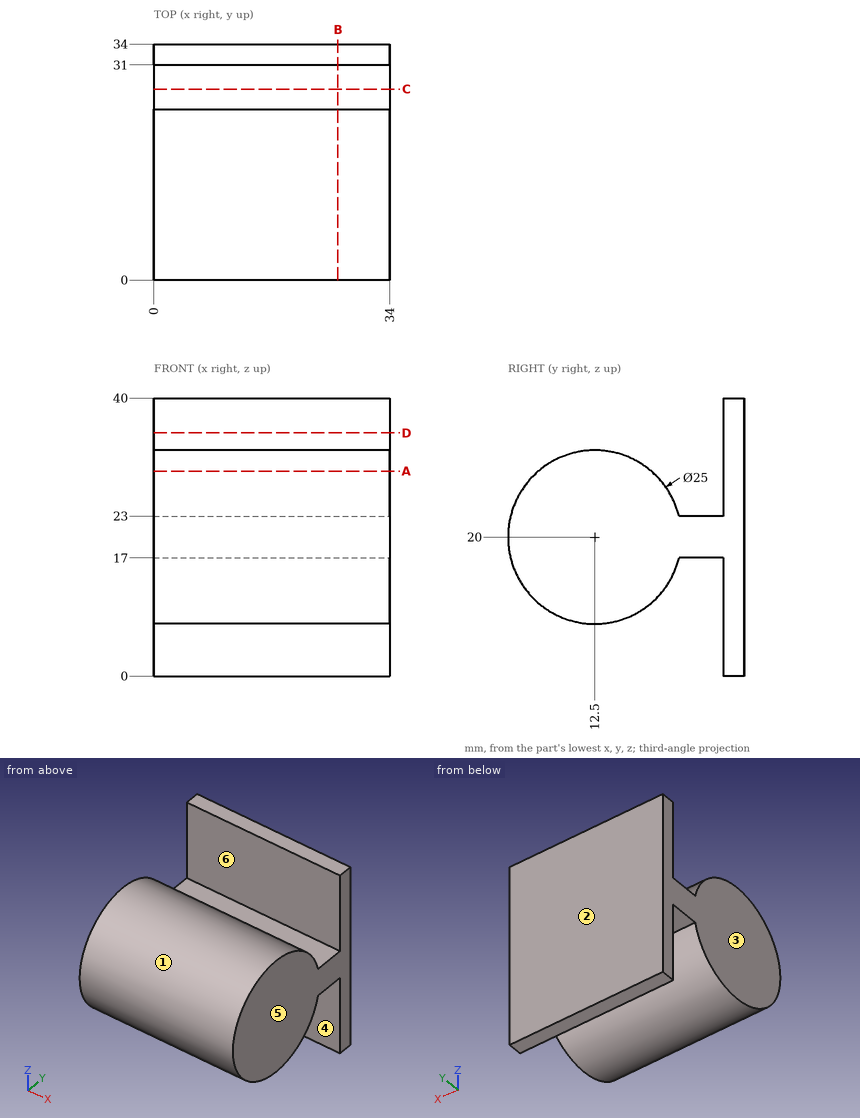
The drawing under review shows one solid part. Ordinate dimensions are in mm from its lowest x, y, z. A direction names the side the tool comes from. Round coordinates to 2 decimals unless told otherwise and drop trailing zeros. Write each loop counter-clockwise with the first axis right and the second up, starting at its lowest first coordinate (ties: lowest second). Pieces come first, ordered by that corner, then holes. Notation, with made-up numbers: (36, 17.5) - (83, 17.5) arc R25 ccw to (83, 55.5) - close; hole circle Ø7 at (-23, 51). An arc over 180 degrees is marked (long way). Put each result on its own line as item: value.
Q1. We need section A-A (z = 29.5). Give the boundary of the cut face in (x, y).
Solved:
outline: (0, 4.38) - (34, 4.38) - (34, 20.62) - (0, 20.62) - close; (0, 31) - (34, 31) - (34, 34) - (0, 34) - close
Q2. We need section D-D (z = 35). Give the boundary of the cut face in (x, y), and give its area (3 significant figures).
Solved:
outline: (0, 31) - (34, 31) - (34, 34) - (0, 34) - close
area: 102 mm2
Q3. Wall thickness on probe 1 along Y at (x, z) = (23.5, 5.5); probe 2 along Z at (x, y) = (2, 29); probe 3 along Z at (x, y) = (16, 13): over which ranges is each line inside the solid? List them lowest first.
Solved:
probe 1: y = 31 to 34
probe 2: z = 17 to 23
probe 3: z = 7.51 to 32.49
Q4. Machinability: for the marked faces 5 and 6, which of the approach directions +Z, -Z, +X, -X, +Y, -Y give a long, thin tool a straight path to every point of the face, cutting with its end or side? Answer none if there is none.
Solved:
face 5: +Z, -Z, +X, +Y, -Y
face 6: +Z, +X, -X
Q5. We need section C-C (y = 27.5). Give the boundary of the cut face in (x, z), and give its area (3 significant figures).
Solved:
outline: (0, 17) - (34, 17) - (34, 23) - (0, 23) - close
area: 204 mm2
Q6. Mouldability with a two-part tool opening along Y and no side actions: class the marked faces 1, 2, 3 and 4 as released by +Y, released by -Y, zero draft, split by the parting line, or undercut.
Solved:
face 1: undercut
face 2: released by +Y
face 3: zero draft
face 4: undercut
Q7. We need section B-B (x = 26.5). Give the boundary of the cut face in (y, z).
Solved:
outline: (24.63, 17) - (31, 17) - (31, 0) - (34, 0) - (34, 40) - (31, 40) - (31, 23) - (24.63, 23) arc R12.5 ccw (long way) to start
Q8. Insertion check: pin 1 Ø13.5 at (x, z) = (14, 7.5) entering from -Y; pin 2 Ø5 at (x, z) = (5, 10.5) entering from -Y; pin 3 Ø3 at (x, y) = (17.5, 11) entering from +Z; pin 4 Ø7 at (x, y) = (24.5, 28) entering from +Z. Each pin has a flat end and moves straight along its axis. Give the tip position at first contact, or say it passes through.
Solved:
pin 1: stops at y = 1.4
pin 2: stops at y = 2.14
pin 3: stops at z = 32.5
pin 4: stops at z = 40
